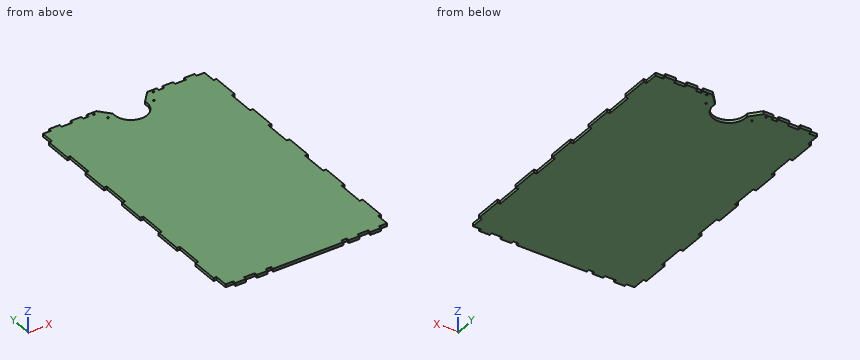
from build123d import *

# Parameters (mm, degrees)
SKETCH_1_W          = 310
SKETCH_1_H          = 510
EXTRUDE_1_DEPTH     = 5.5
SKETCH_2_W          = 5.5
SKETCH_2_H          = 50
CUT_EXTRUDE_1_DEPTH = 299.463146804
CUT_EXTRUDE_2_DEPTH = 299.463146804
SKETCH_5_R          = 1.6
CUT_EXTRUDE_3_DEPTH = 299.463146804
SKETCH_6_R          = 1.55
CUT_EXTRUDE_4_DEPTH = 299.463146804
SKETCH_7_W          = 20
SKETCH_7_H          = 5.5
SKETCH_7_W_2        = 10
CUT_EXTRUDE_5_DEPTH = 299.463146804


with BuildPart() as part:
    # ｽｹｯﾁ1 → ﾎﾞｽ - 押し出し1 (new body)
    with BuildSketch(Plane.XY):
        Rectangle(SKETCH_1_W, SKETCH_1_H)
    extrude(amount=EXTRUDE_1_DEPTH)

    # ｽｹｯﾁ2 → ｶｯﾄ - 押し出し1 (cut, through all)
    with BuildSketch(Plane.XY.offset(5.5)):
        with Locations((152.25, 50)):
            Rectangle(SKETCH_2_W, SKETCH_2_H)
        with Locations((152.25, -50)):
            Rectangle(SKETCH_2_W, SKETCH_2_H)
        with Locations((152.25, 150)):
            Rectangle(SKETCH_2_W, SKETCH_2_H)
        with Locations((152.25, -150)):
            Rectangle(SKETCH_2_W, SKETCH_2_H)
        with Locations((152.25, 250)):
            Rectangle(SKETCH_2_W, SKETCH_2_H)
        with Locations((152.25, -250)):
            Rectangle(SKETCH_2_W, SKETCH_2_H)
        with Locations((-152.25, 50)):
            Rectangle(SKETCH_2_W, SKETCH_2_H)
        with Locations((-152.25, -50)):
            Rectangle(SKETCH_2_W, SKETCH_2_H)
        with Locations((-152.25, 150)):
            Rectangle(SKETCH_2_W, SKETCH_2_H)
        with Locations((-152.25, -150)):
            Rectangle(SKETCH_2_W, SKETCH_2_H)
        with Locations((-152.25, 250)):
            Rectangle(SKETCH_2_W, SKETCH_2_H)
        with Locations((-152.25, -250)):
            Rectangle(SKETCH_2_W, SKETCH_2_H)
    extrude(amount=-CUT_EXTRUDE_1_DEPTH, mode=Mode.SUBTRACT)

    # ｽｹｯﾁ3 → ｶｯﾄ - 押し出し2 (cut, through all)
    with BuildSketch(Plane.XY.offset(5.5)):
        with BuildLine():
            Line((47.033321686, 255), (29.580398915, 235))
            ThreePointArc((29.580398915, 235), (0, 200), (-29.580398915, 235))
            Line((-29.580398915, 235), (-47.033321686, 255))
            Line((-47.033321686, 255), (47.033321686, 255))
        make_face()
    extrude(amount=-CUT_EXTRUDE_2_DEPTH, mode=Mode.SUBTRACT)

    # ｽｹｯﾁ5 → ｶｯﾄ - 押し出し3 (cut, through all)
    with BuildSketch(Plane.XY.offset(5.5)):
        with Locations((-42.5, 230)):
            Circle(SKETCH_5_R)
        with Locations((42.5, 230)):
            Circle(SKETCH_5_R)
    extrude(amount=-CUT_EXTRUDE_3_DEPTH, mode=Mode.SUBTRACT)

    # ｽｹｯﾁ6 → ｶｯﾄ - 押し出し4 (cut, through all)
    with BuildSketch(Plane.XY.offset(5.5)):
        with Locations((55, 250)):
            Circle(SKETCH_6_R)
        with Locations((-55, 250)):
            Circle(SKETCH_6_R)
    extrude(amount=-CUT_EXTRUDE_4_DEPTH, mode=Mode.SUBTRACT)

    # ｽｹｯﾁ7 → ｶｯﾄ - 押し出し5 (cut, through all)
    with BuildSketch(Plane.XY.offset(5.5)):
        with Locations((145, 252.25)):
            Rectangle(SKETCH_7_W, SKETCH_7_H)
        with Locations((105, 252.25)):
            Rectangle(SKETCH_7_W, SKETCH_7_H)
        with Locations((70, 252.25)):
            Rectangle(SKETCH_7_W_2, SKETCH_7_H)
        with Locations((-70, 252.25)):
            Rectangle(SKETCH_7_W_2, SKETCH_7_H)
        with Locations((-105, 252.25)):
            Rectangle(SKETCH_7_W, SKETCH_7_H)
        with Locations((-145, 252.25)):
            Rectangle(SKETCH_7_W, SKETCH_7_H)
        with Locations((-145, -252.25)):
            Rectangle(SKETCH_7_W, SKETCH_7_H)
        with Locations((-105, -252.25)):
            Rectangle(SKETCH_7_W, SKETCH_7_H)
        with Locations((-70, -252.25)):
            Rectangle(SKETCH_7_W_2, SKETCH_7_H)
        with Locations((70, -252.25)):
            Rectangle(SKETCH_7_W_2, SKETCH_7_H)
        with Locations((105, -252.25)):
            Rectangle(SKETCH_7_W, SKETCH_7_H)
        with Locations((145, -252.25)):
            Rectangle(SKETCH_7_W, SKETCH_7_H)
    extrude(amount=-CUT_EXTRUDE_5_DEPTH, mode=Mode.SUBTRACT)


solid = part.part
Model file for the job. Use its own axes, mm. Round coordinates to 2 decimals unless told otherwise and drop trailing zeros. Loops run counter-clockwise (first coordinate to the right, second up) from the corner with the lowest first, then second, coordinate; pieces in that order, holes last. Notation, with made-up numbers: M -30,29.5 L -10,29.5 A24 ccw -10,53.5 Z; hole C 10.5,22.25 d2. An arc over 180 degrees is marked long. One line per question, with ' | ' between items.
1) Flat gauge pins, fed straight in: pin 1 (2 mm diameter, centred on y = -164, z = 4.5, fed in from -X); pin 2 (3 mm diameter, centred on x = -107.5, z = 1.5, fed in from -Y); pin 3 (1.6 mm diameter, centred on y = -251, z = 3.5, fed in from +X); pin 4 (1.9 mm diameter, centred on x = 55, y = 250, fed in from +Z). Where does each tip first touch, or does it go through?
Solved:
pin 1: stops at x = -149.5 | pin 2: stops at y = -249.5 | pin 3: stops at x = 135 | pin 4: passes through
2) Band-saw the part on B-B (y = 156.5). Give the cut face in (x, z).
Solved:
outline: M -149.5,0 L 149.5,0 L 149.5,5.5 L -149.5,5.5 Z
3) Band-saw the part on A-A (x = 0). Give the cut face in (y, z).
Solved:
outline: M -255,0 L 200,0 L 200,5.5 L -255,5.5 Z
4) Band-saw the part on C-C (z = 3.45). Give the number of separate pieces and of enclosed holes in the cut face, then the cut area to 3 significant figures.
Solved:
separate pieces: 1 | enclosed holes: 4 | area: 151,000 mm²
5) Drill centre lines: line 1 along X through (y, z) = (230, 2.6); line 2 along Y through (x, z) = (55, 3); line 3 along X through (y, z) = (-67, 1.05). Where is each one in solid material? Low to high.
Solved:
line 1: x = -149.5 to -44.1, -40.9 to -30, 30 to 40.9, 44.1 to 149.5 | line 2: y = -255 to 248.45, 251.55 to 255 | line 3: x = -149.5 to 149.5
